Source: CAD feature listing. Evaluate the final solid. Frame: model axes, mm. A direction names the side the tool comes from. Give positions to 0.01 mm unless a question says otherwise; leave off trailing zeros. Write each loop counter-clockwise with the first axis right and the second up, starting at its lowest first coordinate (ties: lowest second). Pieces come first, ordered by that corner, then holes. Notation, with made-up numbers: (40.5, -30.5) - (84.5, -30.5) arc R12 cw to (84.5, -11.5) - close; hole circle Ø9 at (22, -4.75). An arc over 180 degrees is marked (long way). Answer as a JSON object with one key per item and string values. Group by question number.
from build123d import *

# Parameters (mm, degrees)
EXTRUDE_1_DEPTH = 100


with BuildPart() as part:
    # 草图1 → 凸台-拉伸1 (new body)
    with BuildSketch(Plane.XY):
        Polygon((-12.227051006, -6.257565337), (-15.227051006, -6.257565337), (-15.227051006, 1.742434663), (-12.227051006, 1.742434663), (-12.227051006, 4.742434663), (-4.027051006, 4.742434663), (-4.027051006, 1.742434663), (-1.027051006, 1.742434663), (-1.027051006, -6.257565337), (-4.027051006, -6.257565337), (-4.027051006, -9.257565337), (31.872948994, -9.257565337), (31.872948994, -3.307565337), (28.872948994, -3.307565337), (28.872948994, -6.307565337), (21.872948994, -6.307565337), (21.872948994, 7.792434663), (28.872948994, 7.792434663), (28.872948994, 4.792434663), (31.872948994, 4.792434663), (31.872948994, 10.742434663), (15.972948994, 10.742434663), (15.972948994, 7.742434663), (18.972948994, 7.742434663), (18.972948994, -0.257565337), (15.972948994, -0.257565337), (15.972948994, -3.257565337), (7.772948994, -3.257565337), (7.772948994, -0.257565337), (4.772948994, -0.257565337), (4.772948994, 7.742434663), (7.772948994, 7.742434663), (7.772948994, 10.742434663), (-24.027051006, 10.742434663), (-24.027051006, 7.742434663), (-21.027051006, 7.742434663), (-21.027051006, -0.257565337), (-24.027051006, -0.257565337), (-24.027051006, -3.257565337), (-32.227051006, -3.257565337), (-32.227051006, -0.257565337), (-35.227051006, -0.257565337), (-35.227051006, 7.742434663), (-32.227051006, 7.742434663), (-32.227051006, 10.742434663), (-48.127051006, 10.742434663), (-48.127051006, 4.792434663), (-45.127051006, 4.792434663), (-45.127051006, 7.792434663), (-38.127051006, 7.792434663), (-38.127051006, -6.307565337), (-45.127051006, -6.307565337), (-45.127051006, -3.307565337), (-48.127051006, -3.307565337), (-48.127051006, -9.257565337), (-12.227051006, -9.257565337), align=None)
    extrude(amount=EXTRUDE_1_DEPTH)


solid = part.part
Q1. Ray query, probe 1 along X at (y, z) = (5, 15); probe 2 along X at (y, z) = (-3, 39); probe 3 along X at (y, z) = (-3.75, 37). Return the intervals inside material, ascending. Write a range as [from, to].
Q2. Section C-C on y = 6.5. Return the cut outline in (x, z), then the cut area to 3 significant figures.
Q3. Section B-B on x = 27. Return the cut outline in (y, z), then the cut area to 3 significant figures.
Q4. Section D-D on x = -30. Return the cut outline in (y, z), then the cut area to 3 significant figures.
Q5. Section A-A on y = -7.75. Return the cut outline in (x, z), then the cut area to 3 significant figures.
Q6. Draft query along Y for faces 1 (the flat face through (-4.027, 3, 49)), 2 (the flat face through (12, -3.258, 49)), 3 (the flat face through (-42, 7.792, 49)). Return one class per face: released by +Y, released by -Y, zero draft, split by the parting line, or undercut.
Q7. First-contact query: pin 1 Ø2.5 at (y, z) = (3.5, 42) entering from +X; pin 2 Ø5 at (x, z) = (10.5, 71) entering from +Y; pin 3 Ø2 at (y, z) = (2, 69.5) entering from -X. Flat tips, straight axial feed; report the tip coordinate or a pass-through.
Q8. Reachability of faces 4 (the flat face through (-42, -6.308, 49)), 5 (the flat face through (14, -9.258, 49)), 6 (the flat face through (-47, -3.308, 49)), 7 (the flat face through (15.973, -2, 49)) from +Z, -Z, +X, -X, +Y, -Y: full face, straight path, thin tool, end or side. Return the list, or none.
Taken from the geometry:
{
 "1": {"probe 1": "x = [-48.13, -45.13], [-38.13, -35.23], [-21.03, 4.77], [18.97, 21.87], [28.87, 31.87]", "probe 2": "x = [-38.13, -32.23], [-24.03, -15.23], [-1.03, 7.77], [15.97, 21.87]", "probe 3": "x = [-48.13, -45.13], [-38.13, -15.23], [-1.03, 21.87], [28.87, 31.87]"},
 "2": {"outline": "(-48.13, 0) - (-45.13, 0) - (-45.13, 100) - (-48.13, 100) - close; (-38.13, 0) - (-35.23, 0) - (-35.23, 100) - (-38.13, 100) - close; (-21.03, 0) - (4.77, 0) - (4.77, 100) - (-21.03, 100) - close; (18.97, 0) - (21.87, 0) - (21.87, 100) - (18.97, 100) - close; (28.87, 0) - (31.87, 0) - (31.87, 100) - (28.87, 100) - close", "area": "3,760 mm²"},
 "3": {"outline": "(-9.26, 0) - (-6.31, 0) - (-6.31, 100) - (-9.26, 100) - close; (7.79, 0) - (10.74, 0) - (10.74, 100) - (7.79, 100) - close", "area": "590 mm²"},
 "4": {"outline": "(-9.26, 0) - (-3.26, 0) - (-3.26, 100) - (-9.26, 100) - close", "area": "600 mm²"},
 "5": {"outline": "(-48.13, 0) - (-12.23, 0) - (-12.23, 100) - (-48.13, 100) - close; (-4.03, 0) - (31.87, 0) - (31.87, 100) - (-4.03, 100) - close", "area": "7,180 mm²"},
 "6": {"face 1": "zero draft", "face 2": "released by +Y", "face 3": "undercut"},
 "7": {"pin 1": "stops at x = 21.87", "pin 2": "stops at y = -3.26", "pin 3": "stops at x = -38.13"},
 "8": {"face 4": "+Z, -Z", "face 5": "+Z, -Z, +X, -X, -Y", "face 6": "+Z, -Z, -X", "face 7": "+Z, -Z, +Y"}
}
